```python
from build123d import *

# Parameters (mm, degrees)
SKETCH1_W            = 20
SKETCH1_H            = 6
BOSS_EXTRUDE1_DEPTH  = 20.5
SKETCH2_W            = 3
SKETCH2_H            = 20
BOSS_EXTRUDE2_DEPTH  = 12
SKETCH7_R            = 1.5
CUT_EXTRUDE1_DEPTH   = 44.874821937
SKETCH8_R            = 3.4
CUT_EXTRUDE2_DEPTH   = 30.055980452
FILLET2_R            = 3
CONVERT_SOLID2_START = -10
CONVERT_SOLID2_DEPTH = 20


# Read off the part's stored shape, not the designer's step: Convert-Solid2
with BuildPart() as part:
    # Sketch1 → Boss-Extrude1 (new, symmetric)
    with BuildSketch(Plane(origin=(0, 0, 0), x_dir=(0, 0, -1), z_dir=(1, 0, 0))):
        with Locations((0, -3)):
            Rectangle(SKETCH1_W, SKETCH1_H)
    extrude(amount=BOSS_EXTRUDE1_DEPTH, both=True)

    # Sketch2 → Boss-Extrude2 (add)
    with BuildSketch(Plane(origin=(0, 0, 0), x_dir=(1, 0, 0), z_dir=(0, 1, 0))):
        with Locations((19, 0)):
            Rectangle(SKETCH2_W, SKETCH2_H)
        with Locations((-19, 0)):
            Rectangle(SKETCH2_W, SKETCH2_H)
    extrude(amount=BOSS_EXTRUDE2_DEPTH)

    # Sketch7 → Cut-Extrude1 (cut, through all)
    with BuildSketch(Plane.ZY.offset(20.5)):
        with Locations((-5, 7)):
            Circle(SKETCH7_R)
        with Locations((5, 7)):
            Circle(SKETCH7_R)
    extrude(amount=-CUT_EXTRUDE1_DEPTH, mode=Mode.SUBTRACT)

    # Sketch8 → Cut-Extrude2 (cut, through all)
    with BuildSketch(Plane.XZ.offset(6)):
        with Locations(Location((0, 0, 0), (0, 0, 270))):
            Circle(SKETCH8_R)
    extrude(amount=-CUT_EXTRUDE2_DEPTH, mode=Mode.SUBTRACT)

    # Fillet2
    fillet2_edges = [part.edges().sort_by_distance(p)[0] for p in [
        (-19, 12, 10),
        (-19, 12, -10),
        (19, 12, -10),
        (19, 12, 10),
    ]]
    fillet(fillet2_edges, radius=FILLET2_R)

    # Convert-Solid2 outline → Convert-Solid2 (cut)
    with BuildSketch(Plane.XY.offset(CONVERT_SOLID2_START)):
        with BuildLine():
            Line((20.5, -6), (20.5, 0))
            ThreePointArc((20.5, 0), (18.742640687, -4.242640687), (14.5, -6))
            Line((14.5, -6), (20.5, -6))
        make_face()
        with BuildLine():
            Line((-20.5, -6), (-14.5, -6))
            ThreePointArc((-14.5, -6), (-18.742640687, -4.242640687), (-20.5, 0))
            Line((-20.5, 0), (-20.5, -6))
        make_face()
        with BuildLine():
            Line((18.5, 0), (18.5, 12))
            Line((18.5, 12), (17.5, 12))
            Line((17.5, 12), (17.5, 0))
            Line((17.5, 0), (-17.5, 0))
            Line((-17.5, 0), (-17.5, 12))
            Line((-17.5, 12), (-18.5, 12))
            Line((-18.5, 12), (-18.5, 0))
            ThreePointArc((-18.5, 0), (-17.328427125, -2.828427125), (-14.5, -4))
            Line((-14.5, -4), (14.5, -4))
            ThreePointArc((14.5, -4), (17.328427125, -2.828427125), (18.5, 0))
        make_face()
    extrude(amount=CONVERT_SOLID2_DEPTH, mode=Mode.SUBTRACT)


solid = part.part
```
Geometry check sheet. Reference: the model listing, model coordinates, mm. A direction names the side the tool comes from. Round coordinates to 2 decimals unless told otherwise and drop trailing zeros. Write each loop counter-clockwise with the first axis right and the second up, starting at its lowest first coordinate (ties: lowest second). Pieces come first, ordered by that corner, then holes. Notation, with made-up numbers: (-29.5, -12.5) -> (-2.5, -12.5) arc R18 ccw to (-2.5, 8.5) -> close; hole circle Ø7 at (40, 45). An arc over 180 degrees is marked (long way). Put each result on its own line as item: value.
1) Release check for a two-part mould opening along Y. For faces 1 (the face through (19.486, 5.536, -5.325)), 2 (the face through (19.51, 11.1, 9.14)), 3 (the face through (-19.514, 5.536, -5.325)), 4 (the face through (20.5, 6, 0)) record: pulls with the +Y half, pulls with the -Y half, needs draft (parallel to the pull), parting line crosses it, or undercut.
Recorded:
face 1: undercut
face 2: pulls with the +Y half
face 3: undercut
face 4: needs draft
2) Cross-section at D-D, the plane z = -1.75. Enter the section's corners in (x, y), plus the area to 3 significant figures.
Recorded:
outline: (-20.5, 0) arc R6 ccw to (-14.5, -6) -> (-2.92, -6) -> (-2.92, -4) -> (-14.5, -4) arc R4 cw to (-18.5, 0) -> (-18.5, 12) -> (-20.5, 12) -> close; (2.92, -6) -> (14.5, -6) arc R6 ccw to (20.5, 0) -> (20.5, 12) -> (18.5, 12) -> (18.5, 0) arc R4 cw to (14.5, -4) -> (2.92, -4) -> close
area: 126 mm2
3) Access from +Z, -Z, +X, -X, +Y, -Y to the whole of each face (thin tool, end or side, straight path). Record for faces 5 (the face through (-18.696, -4.289, -0.14)), 6 (the face through (17.297, -2.859, -0.14)).
Recorded:
face 5: +Z, -Z, -X, -Y
face 6: +Z, -Z, +Y
4) Depth check by flat-ended pin: P1, Ø8, axis at x = -1, z = -4, coming from the +Y side; P2, Ø6, axis at x = 0, z = 0, coming from the +Y side; P3, Ø1.5, axis at x = -15.5, z = 6.5, coming from the +Y side. Enter the tip coordinate at first touch or a pass-through.
Recorded:
P1: stops at y = -4
P2: passes through
P3: stops at y = -3.6
5) Cross-section at B-B, the plane z = -5. Enter the section's corners in (x, y), plus the area to 3 significant figures.
Recorded:
outline: (-20.5, 0) arc R6 ccw to (-14.5, -6) -> (14.5, -6) arc R6 ccw to (20.5, 0) -> (20.5, 5.5) -> (18.5, 5.5) -> (18.5, 0) arc R4 cw to (14.5, -4) -> (-14.5, -4) arc R4 cw to (-18.5, 0) -> (-18.5, 5.5) -> (-20.5, 5.5) -> close; (-20.5, 8.5) -> (-18.5, 8.5) -> (-18.5, 12) -> (-20.5, 12) -> close; (18.5, 8.5) -> (20.5, 8.5) -> (20.5, 12) -> (18.5, 12) -> close
area: 125 mm2
6) Thickness scan on probe 1 along X at (y, z) = (4.25, -7.5); probe 2 along Y at (x, z) = (9, 6.5); probe 3 along X at (y, z) = (-1.75, -2.75). Record the ranges inside material, lowest first. Write a range as from..to.
Recorded:
probe 1: x = -20.5..-18.5, 18.5..20.5
probe 2: y = -6..-4
probe 3: x = -20.24..-18.1, 18.1..20.24
7) Cross-section at C-C, the plane y = -3.5. Enter the section's corners in (x, z), plus the area to 3 significant figures.
Recorded:
outline: (-19.37, -10) -> (-16.44, -10) -> (-16.44, 10) -> (-19.37, 10) -> close; (16.44, -10) -> (19.37, -10) -> (19.37, 10) -> (16.44, 10) -> close
area: 117 mm2
8) Cross-section at A-A, the plane y = 7. Enter the section's corners in (x, z), plus the area to 3 significant figures.
Recorded:
outline: (-20.5, -10) -> (-18.5, -10) -> (-18.5, -6.5) -> (-20.5, -6.5) -> close; (-20.5, -3.5) -> (-18.5, -3.5) -> (-18.5, 3.5) -> (-20.5, 3.5) -> close; (-20.5, 6.5) -> (-18.5, 6.5) -> (-18.5, 10) -> (-20.5, 10) -> close; (18.5, -10) -> (20.5, -10) -> (20.5, -6.5) -> (18.5, -6.5) -> close; (18.5, -3.5) -> (20.5, -3.5) -> (20.5, 3.5) -> (18.5, 3.5) -> close; (18.5, 6.5) -> (20.5, 6.5) -> (20.5, 10) -> (18.5, 10) -> close
area: 56.0 mm2
